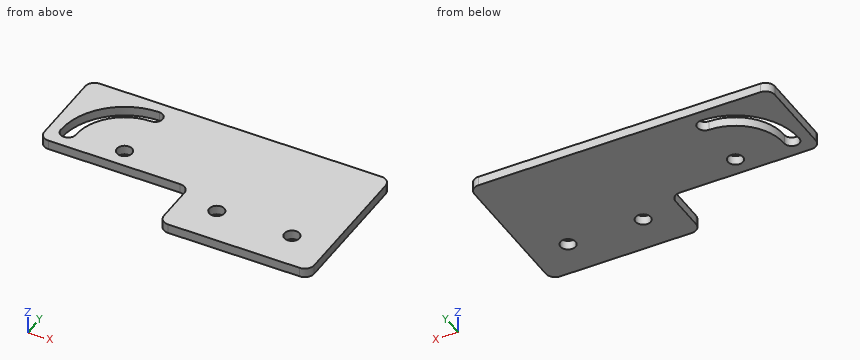
```python
from build123d import *

# Parameters (mm, degrees)
SKETCH1_W           = 50.8
SKETCH1_H           = 50.8
SKETCH1_R           = 2.5527
SKETCH1_H_2         = 31.75
BOSS_EXTRUDE1_DEPTH = 3.175
FILLET1_R           = 3.175


with BuildPart() as part:
    # Sketch1 → Boss-Extrude1 (new body)
    # profile 1 of 2: a face of its own
    with BuildSketch(Plane.XY):
        with Locations((25.4, 25.4)):
            Rectangle(SKETCH1_W, SKETCH1_H)
        with Locations((38.1, 12.7)):
            Circle(SKETCH1_R, mode=Mode.SUBTRACT)
        with Locations((12.7, 12.7)):
            Circle(SKETCH1_R, mode=Mode.SUBTRACT)
    # profile 2 of 2: a face of its own
    with BuildSketch(Plane.XY):
        with Locations((-25.4, 34.925)):
            Rectangle(SKETCH1_W, SKETCH1_H_2)
        with Locations((-25.4, 25.4)):
            Circle(SKETCH1_R, mode=Mode.SUBTRACT)
        with BuildLine():
            ThreePointArc((-41.8973, 25.4), (-44.45, 22.8473), (-47.0027, 25.4))
            ThreePointArc((-47.0027, 25.4), (-40.675415662, 40.675415662), (-25.4, 47.0027))
            ThreePointArc((-25.4, 47.0027), (-22.8473, 44.45), (-25.4, 41.8973))
            ThreePointArc((-25.4, 41.8973), (-37.065352701, 37.065352701), (-41.8973, 25.4))
        make_face(mode=Mode.SUBTRACT)
    extrude(amount=BOSS_EXTRUDE1_DEPTH)

    # Fillet1
    fillet1_edges = [part.edges().sort_by_distance(p)[0] for p in [
        (0, 0, 1.5875),
        (0, 19.05, 1.5875),
        (-50.8, 19.05, 1.5875),
        (-50.8, 50.8, 1.5875),
        (50.8, 50.8, 1.5875),
        (50.8, 0, 1.5875),
    ]]
    fillet(fillet1_edges, radius=FILLET1_R)


solid = part.part
```
Geometry: final body of the model. Coordinates: model frame, mm. Give positions to 0.01 mm unless a question says otherwise; leave off trailing zeros. Order: outer loops, then holes, each group sorted by start corner. A loop starts at its lowest first (then second) coordinate and runs counter-clockwise, first axis right, second up. Notation, with made-up numbers: M 38,41 L 44,41 A13 ccw 44,57 Z; hole C 61,10.5 d8. An arc over 180 degrees is marked long. Answer as CSV lines item,"result". Start each with the question number.
1) First-contact query: P1, Ø1, axis at x = -17.5, z = 1, coming from the -Y side. Flat tip, straight axial feed; report the tip coordinate or a pass-through.
2) Line query: line 1 (Y direction, x = -25.4, z = 0.7); line 2 (Y direction, x = 38.1, z = 2); line 3 (Y direction, x = -8, z = 2.25). Output: solid intervals per line, ascending. Write a range as from..to.
3) Cut plane B-B (z = 1.85). Output: boundary loops of the cut face in (x, y) (3 decimals).
4) Cut plane A-A (x = 38.1). Output: boundary loops of the cut face in (y, z) (3 decimals).
5) Cut plane C-C (y = 34). Output: boundary loops of the cut face in (x, z) (3 decimals).
6) Cut plane D-D (x = -27). Output: boundary loops of the cut face in (y, z) (3 decimals).
Findings below:
1,P1,"stops at y = 19.05"
2,line 1,"y = 19.05..22.85, 27.95..41.9, 47..50.8"
2,line 2,"y = 0..10.15, 15.25..50.8"
2,line 3,"y = 19.05..50.8"
3,outline,"M -50.8,22.225 A3.175 ccw -47.625,19.05 L -3.175,19.05 A3.175 cw 0,15.875 L 0,3.175 A3.175 ccw 3.175,0 L 47.625,0 A3.175 ccw 50.8,3.175 L 50.8,47.625 A3.175 ccw 47.625,50.8 L -47.625,50.8 A3.175 ccw -50.8,47.625 Z; hole M -47.003,25.4 A2.553 ccw -41.897,25.4 A16.497 cw -25.4,41.897 A2.553 ccw -25.4,47.003 A21.603 ccw Z; hole C -25.4,25.4 d5.105; hole C 12.7,12.7 d5.105; hole C 38.1,12.7 d5.105"
4,outline,"M 0,0 L 10.147,0 L 10.147,3.175 L 0,3.175 Z; M 15.253,0 L 50.8,0 L 50.8,3.175 L 15.253,3.175 Z"
5,outline,"M -50.8,0 L -45.217,0 L -45.217,3.175 L -50.8,3.175 Z; M -39.478,0 L 50.8,0 L 50.8,3.175 L -39.478,3.175 Z"
6,outline,"M 19.05,0 L 23.411,0 L 23.411,3.175 L 19.05,3.175 Z; M 27.389,0 L 41.82,0 L 41.82,3.175 L 27.389,3.175 Z; M 46.943,0 L 50.8,0 L 50.8,3.175 L 46.943,3.175 Z"
